Verification items for the finished model (mm, model axes). Face numbers are marked on the shaded views. A direction names the side the tool comes from. Coordinates: 2 decimals unless noted, no trailing zeros. Write each loop counter-clockwise with the first axis right and the second up, starting at its lowest first coordinate (ties: lowest second). Pieces come first, ordered by that corner, then holes. Notation, with made-up numbers: (-37, -33) - (8, -33) arc R24 ccw to (8, -11) - close; hole circle Ø8 at (16.25, 84.5). An arc over 180 degrees is marked (long way). Answer as CSV lines item,"result". Start each with the question number.
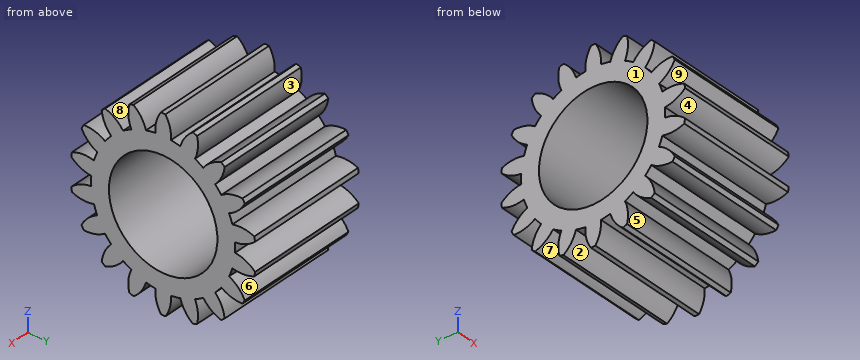
```python
from build123d import *

# Parameters (mm, degrees)
BASPROSKE_W        = 8
BASPROSKE_H        = 6
TOOTHCUT_DEPTH     = 12.66190379
TEETHCUTS_COUNT    = 18
TEETHCUTS_ANGLE    = 340
BORSKE_R           = 0.5
BORE_DEPTH         = 50.0000508
SKETCH1_R          = 3.5
CUT_EXTRUDE1_DEPTH = 12.627390673


with BuildPart() as part:
    # BasProSke → Base-Revolve (revolve)
    with BuildSketch(Plane(origin=(0, 0, 0), x_dir=(1, 0, 0), z_dir=(0, 1, 0)), mode=Mode.PRIVATE) as base_revolve_sk:
        with Locations((4, 3)):
            Rectangle(BASPROSKE_W, BASPROSKE_H)
    revolve(base_revolve_sk.sketch.rotate(Axis((-10, 0, 0), (1, 0, 0)), 180), axis=Axis((-10, 0, 0), (1, 0, 0)))

    # TooCutSke → ToothCut (cut, through all)
    with BuildSketch(Plane(origin=(0, 0, 0), x_dir=(0, 0, -1), z_dir=(1, 0, 0))):
        with BuildLine():
            ThreePointArc((0.306649621, 4.638875619), (0, 4.649), (-0.306649621, 4.638875619))
            ThreePointArc((-0.306649621, 4.638875619), (-0.498605842, 5.349852231), (-0.918258882, 5.955018538))
            ThreePointArc((-0.918258882, 5.955018538), (0, 6.0254), (0.918258882, 5.955018538))
            ThreePointArc((0.918258882, 5.955018538), (0.498605842, 5.349852231), (0.306649621, 4.638875619))
        make_face()
    toothcut = extrude(amount=TOOTHCUT_DEPTH, mode=Mode.SUBTRACT)

    # TeethCuts: ToothCut ×18 about axis
    teethcuts_axis = Axis((-10, 0, 0), (1, 0, 0))
    for i in range(1, TEETHCUTS_COUNT):
        add(toothcut.rotate(teethcuts_axis, i * TEETHCUTS_ANGLE / (TEETHCUTS_COUNT - 1)), mode=Mode.SUBTRACT)

    # BorSke → Bore (cut, symmetric)
    with BuildSketch(Plane(origin=(0, 0, 0), x_dir=(0, 0, -1), z_dir=(1, 0, 0))):
        with Locations(Location((0, 0, 0), (0, 0, 180))):
            Circle(BORSKE_R)
    extrude(amount=BORE_DEPTH, both=True, mode=Mode.SUBTRACT)

    # Sketch1 → Cut-Extrude1 (cut, through all)
    with BuildSketch(Plane(origin=(8, 0, 0), x_dir=(0, 0, -1), z_dir=(1, 0, 0))):
        Circle(SKETCH1_R)
    extrude(amount=-CUT_EXTRUDE1_DEPTH, mode=Mode.SUBTRACT)


solid = part.part
```
1. Depth check by flat-ended pin: P1, Ø2, axis at x = 2.5, z = 3.5, coming from the +Y side; P2, Ø2, axis at x = 3, y = -3.5, coming from the -Z side; P3, Ø2, axis at x = 3.5, z = 1.5, coming from the -Y side. Enter the tip coordinate at first touch or a pass-through.
2. Draft check along Z on the marked faces 1, 2, 3 and 4. Enter one of: pulls with the +Z half, pulls with the -Z half, needs draft (parallel to the pull), parting line crosses it, or undercut.
3. Scan lines: line 1 along Z through (x, y) = (2, -5); line 2 along Y through (x, z) = (4.5, 0); line 3 along Y through (x, z) = (6.75, 4.75). Record each from-to range of solid material in increasing order. Write a range as from..to.
4. Cross-section at A-A (z = 0). Record the cut outline in (x, y), and give its area (3 significant figures).
5. Access from +Z, -Z, +X, -X, +Y, -Y to the whole of each face (thin tool, end or side, straight path). Record for the marked faces 5, 6, 7, 8 and 9.
6. Cross-section at B-B (y = 2.75). Record the cut outline in (x, z).
Completed:
1,P1,"stops at y = 5.27"
1,P2,"stops at z = -4.69"
1,P3,"stops at y = -5.93"
2,face 1,"needs draft"
2,face 2,"pulls with the -Z half"
2,face 3,"undercut"
2,face 4,"undercut"
3,line 1,"z = -3.13..-2.46, -1.37..-0.37, 0.37..1.37, 2.46..3.13"
3,line 2,"y = -4.65..-3.5, 3.5..4.65"
3,line 3,"y = -2.23..-1.19, -0.51..0.51, 1.19..2.23"
4,outline,"(0, -4.65) - (8, -4.65) - (8, -3.5) - (0, -3.5) - close; (0, 3.5) - (8, 3.5) - (8, 4.65) - (0, 4.65) - close"
4,area,"18.4 mm2"
5,face 5,"+X, -X"
5,face 6,"+X, -X, +Y"
5,face 7,"-Z, +X, -X"
5,face 8,"+Z, +X, -X"
5,face 9,"+X, -X, -Y"
6,outline,"(0, -4.07) - (8, -4.07) - (8, -2.17) - (0, -2.17) - close; (0, 2.17) - (8, 2.17) - (8, 4.07) - (0, 4.07) - close"
